```python
from build123d import *

# Parameters (mm, degrees)
F0_W      = 154
F0_H      = 78
F1_DEPTH  = 46.5
F3_DEPTH  = 80
F4_R      = 7.5
F5_DEPTH  = 50
F6_R      = 29
F7_DEPTH  = 30
F8_SIZE2  = 3.99999
F8_SIZE   = 29.99999
F9_R      = 7.5
F10_DEPTH = 40


# Not quite as in the source:
# - a fillet or chamfer is up to 0.001 mm smaller than in the source, because OpenCascade refuses the exact size


with BuildPart() as f1:
    # F0 (on Top) → F1 (new body, symmetric)
    with BuildSketch(Plane.XY):
        Rectangle(F0_W, F0_H)
    extrude(amount=F1_DEPTH, both=True)

    # F2 (on face) → F3 (cut)
    with BuildSketch(Plane.XZ.offset(39)):
        Polygon((-77, 46.5), (-77, -13.5), (-42.5, -13.5), (-27.0954341594, 8.5), (-58, 8.5), (-58, 46.5), align=None)
        Polygon((77, 46.5), (58, 46.5), (58, 8.5), (27.0954341594, 8.5), (42.5, -13.5), (77, -13.5), align=None)
    extrude(amount=-F3_DEPTH, mode=Mode.SUBTRACT)

    # F4 (on face) → F5 (cut)
    with BuildSketch(Plane.XY.offset(-13.5)):
        with Locations((-67.5, 0)):
            Circle(F4_R)
    extrude(amount=-F5_DEPTH, mode=Mode.SUBTRACT)

    # F6 (on face) → F7 (cut)
    with BuildSketch(Plane.XY.offset(46.5)):
        Circle(F6_R)
    extrude(amount=-F7_DEPTH, mode=Mode.SUBTRACT)

    # F8 (size 30 and 4 in the source; OpenCascade refuses exactly that, so slightly less here)
    f8_edges = [f1.edges().sort_by_distance(p)[0] for p in [
        (-29, 0, 16.5),
    ]]
    f8_side = f1.faces().sort_by_distance((-29, 0, 31.5))[0]
    chamfer(f8_edges, length=F8_SIZE, length2=F8_SIZE2, reference=f8_side)

    # F9 (on face) → F10 (cut)
    with BuildSketch(Plane.XY.offset(-13.5)):
        with Locations((67.5, 0)):
            Circle(F9_R)
    extrude(amount=-F10_DEPTH, mode=Mode.SUBTRACT)


solid = f1.part
```
The listing builds one solid part. Answer for the finished solid, in the listing's coordinates (mm). A direction names the side the tool comes from. Coordinates: 2 decimals unless noted, no trailing zeros. Write each loop counter-clockwise with the first axis right and the second up, starting at its lowest first coordinate (ties: lowest second). Pieces come first, ordered by that corner, then holes. Notation, with made-up numbers: (-14.5, 38.25) - (37.5, 38.25) arc R15 cw to (37.5, 42.25) - close; hole circle Ø2 at (19.25, 8.25). An arc over 180 degrees is marked (long way). Return JSON: item names as keys, results as strings. Group by question number.
Q1. Flat-ended cylindrical pins translate along their axes: pin 1 Ø19 at (y, z) = (-15, 32.5) entering from +X; pin 2 Ø1 at (y, z) = (-1.5, -1.5) entering from +X; pin 3 Ø6 at (y, z) = (27, 30.5) entering from -X; pin 4 Ø12 at (x, y) = (-67.5, 0) entering from +Z. Find the tip coordinate at first contact, or state that the pin passes through.
Q2. For a pull along Z with two mould halves and no side action, classify faces 1 (the flat face through (-58, -1, 27)), 2 (the flat face through (59.5, -0.5, -13.5)), 3 (the conical face through (-21.051, -16.142, 27.957)) as +Z half, -Z half, draft (parallel to the pull), parting line (faces both ways), or undercut.
Q3. The part is cut by section B-B on y = 0. State how many separate pieces and enclosed holes the cut face has, and give its area (3 significant figures).
Q4. The part is cut by section A-A on x = -63. Write down the section's boundary in (y, z).
Q5. Which of the six approach directions +Z, -Z, +X, -X, +Y, -Y give full straight-line access (tool end or side, diameter ignored) to faces 4 (the flat face through (-56, -1, -13.5)), 5 (the flat face through (58, -1, 28)), 6 (the flat face through (34.69, -0.546, -2.346)), 7 (the flat face through (0, 0, 16.5))?
Q6. Find the intervals of material crossed by line 1 along Z through (x, y) = (45.5, -13.5); line 2 along X through (y, z) = (-6.5, -36.5); line 3 along Y through (x, z) = (-67.5, -37), in increasing order. Write a range as [from, to].
Q7. The part is cut by section C-C on z = -31. Write down the section's boundary in (x, y), and give its area (3 significant figures).
Evaluation:
{
 "1": {"pin 1": "stops at x = 58", "pin 2": "stops at x = 34.45", "pin 3": "stops at x = -58", "pin 4": "passes through"},
 "2": {"face 1": "draft", "face 2": "undercut", "face 3": "+Z half"},
 "3": {"separate pieces": "3", "enclosed holes": "0", "area": "8,410 mm2"},
 "4": {"outline": "(-39, -46.5) - (-6, -46.5) - (-6, -13.5) - (-39, -13.5) - close; (6, -46.5) - (39, -46.5) - (39, -13.5) - (6, -13.5) - close"},
 "5": {"face 4": "-X, +Y, -Y", "face 5": "+Z, +X, +Y, -Y", "face 6": "+X, +Y, -Y", "face 7": "+Z"},
 "6": {"line 1": "z = [-46.5, -13.5], [8.5, 46.5]", "line 2": "x = [-77, -71.24], [-63.76, 63.76], [71.24, 77]", "line 3": "y = [-39, -7.5], [7.5, 39]"},
 "7": {"outline": "(-77, -39) - (77, -39) - (77, 39) - (-77, 39) - close; hole circle Ø15 at (-67.5, 0); hole circle Ø15 at (67.5, 0)", "area": "11,700 mm2"}
}
